Here's how the part is built. I have some questions about the finished solid (model axes, mm). Face numbers are marked on the shaded views. A direction names the side the tool comes from. Round coordinates to 2 decimals unless told otherwise and drop trailing zeros. Order: outer loops, then holes, each group sorted by start corner. A loop starts at its lowest first (then second) coordinate and runs counter-clockwise, first axis right, second up. Notation, with made-up numbers: M 46.5,48 L 79.5,48 A13 cw 79.5,58 Z; hole C -29.5,-39 d10. An arc over 180 degrees is marked long. Write each question's results on one line, items separated by ' | '. Start each with the question number.
```python
from build123d import *

# Parameters (mm, degrees)
SKETCH1_W           = 76.2
SKETCH1_H           = 25.4
SKETCH1_W_2         = 69.85
SKETCH1_H_2         = 19.05
BOSS_EXTRUDE1_DEPTH = 152.4
SKETCH2_R           = 3.3782
CUT_EXTRUDE1_DEPTH  = 26.4
SKETCH3_R           = 5.0419
CUT_EXTRUDE2_DEPTH  = 26.4


with BuildPart() as part:
    # Sketch1 → Boss-Extrude1 (new body)
    with BuildSketch(Plane.XY):
        with Locations((38.1, 12.7)):
            Rectangle(SKETCH1_W, SKETCH1_H)
        with Locations((38.1, 12.7)):
            Rectangle(SKETCH1_W_2, SKETCH1_H_2, mode=Mode.SUBTRACT)
    extrude(amount=BOSS_EXTRUDE1_DEPTH)

    # Sketch2 → Cut-Extrude1 (cut, through all)
    with BuildSketch(Plane(origin=(0, 25.4, 0), x_dir=(1, 0, 0), z_dir=(0, 1, 0))):
        with Locations((13.21308, -16.2687)):
            Circle(SKETCH2_R)
        with Locations((29.80436, -16.2687)):
            Circle(SKETCH2_R)
        with Locations((46.39564, -16.2687)):
            Circle(SKETCH2_R)
        with Locations((62.98692, -16.2687)):
            Circle(SKETCH2_R)
    extrude(amount=-CUT_EXTRUDE1_DEPTH, mode=Mode.SUBTRACT)

    # Sketch3 → Cut-Extrude2 (cut, through all)
    with BuildSketch(Plane.XZ):
        with Locations((60.325, 139.7)):
            Circle(SKETCH3_R)
        with Locations((15.875, 139.7)):
            Circle(SKETCH3_R)
    extrude(amount=-CUT_EXTRUDE2_DEPTH, mode=Mode.SUBTRACT)


solid = part.part
```
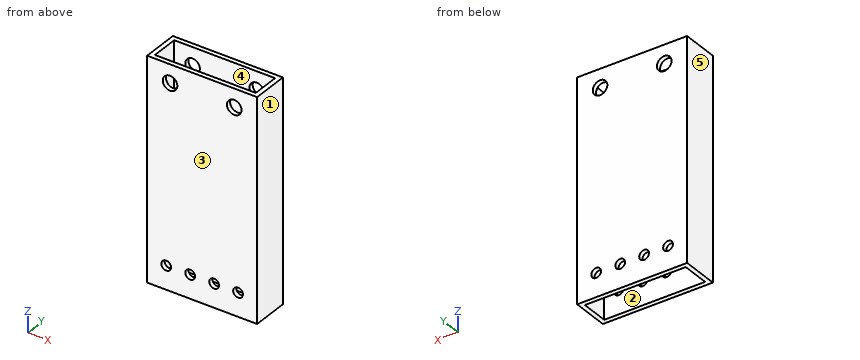
(1) On a 3-axis mill with a long thin cutter (end or side, diameter ignored), from which of +Z, -Z, +X, -X, +Y, -Y can I reach the whole of each face in a straight line? I mean the marked faces 1 and 2. Say none if no direction works.
(2) I want a section at D-D on z = 76. Write out the boundary of the cut face in (x, y) (3 decimals).
(3) If we mould it in two halves opening along X, with no side actions, what happens to the marked faces 3, 4 and 5? For each: pulls with the +X half, pulls with the -X half, needs draft (parallel to the pull), parting line crosses it, or undercut.
(4) Please list where these lines run through material, in increasing order: line 1 (X direction, y = 14, z = 133) (3 decimals); line 2 (Y direction, x = 60, z = 67) (3 decimals); line 3 (Z direction, x = 46, y = 2.5).
(5) I want a section at A-A on y = 16.25. Write out the boundary of the cut face in (x, z) (3 decimals).
(6) I want a section at B-B on x = 39. Write out the boundary of the cut face in (y, z) (3 decimals), and give its area (3 significant figures).
(7) I want a section at C-C on z = 139.7. Write out the boundary of the cut face in (x, y) (3 decimals).
Solutions:
1) face 1: +Z, -Z, +X, +Y, -Y | face 2: +Z, -Z
2) outline: M 0,0 L 76.2,0 L 76.2,25.4 L 0,25.4 Z; hole M 3.175,3.175 L 73.025,3.175 L 73.025,22.225 L 3.175,22.225 Z
3) face 3: needs draft | face 4: undercut | face 5: pulls with the -X half
4) line 1: 0 to 3.175, 73.025 to 76.2 | line 2: 0 to 3.175, 22.225 to 25.4 | line 3: 0 to 12.91, 19.62 to 152.4
5) outline: M 0,0 L 3.175,0 L 3.175,152.4 L 0,152.4 Z; M 73.025,0 L 76.2,0 L 76.2,152.4 L 73.025,152.4 Z
6) outline: M 0,0 L 3.175,0 L 3.175,152.4 L 0,152.4 Z; M 22.225,0 L 25.4,0 L 25.4,152.4 L 22.225,152.4 Z | area: 968 mm^2
7) outline: M 0,0 L 10.833,0 L 10.833,3.175 L 3.175,3.175 L 3.175,22.225 L 10.833,22.225 L 10.833,25.4 L 0,25.4 Z; M 20.917,0 L 55.283,0 L 55.283,3.175 L 20.917,3.175 Z; M 20.917,22.225 L 55.283,22.225 L 55.283,25.4 L 20.917,25.4 Z; M 65.367,0 L 76.2,0 L 76.2,25.4 L 65.367,25.4 L 65.367,22.225 L 73.025,22.225 L 73.025,3.175 L 65.367,3.175 Z
